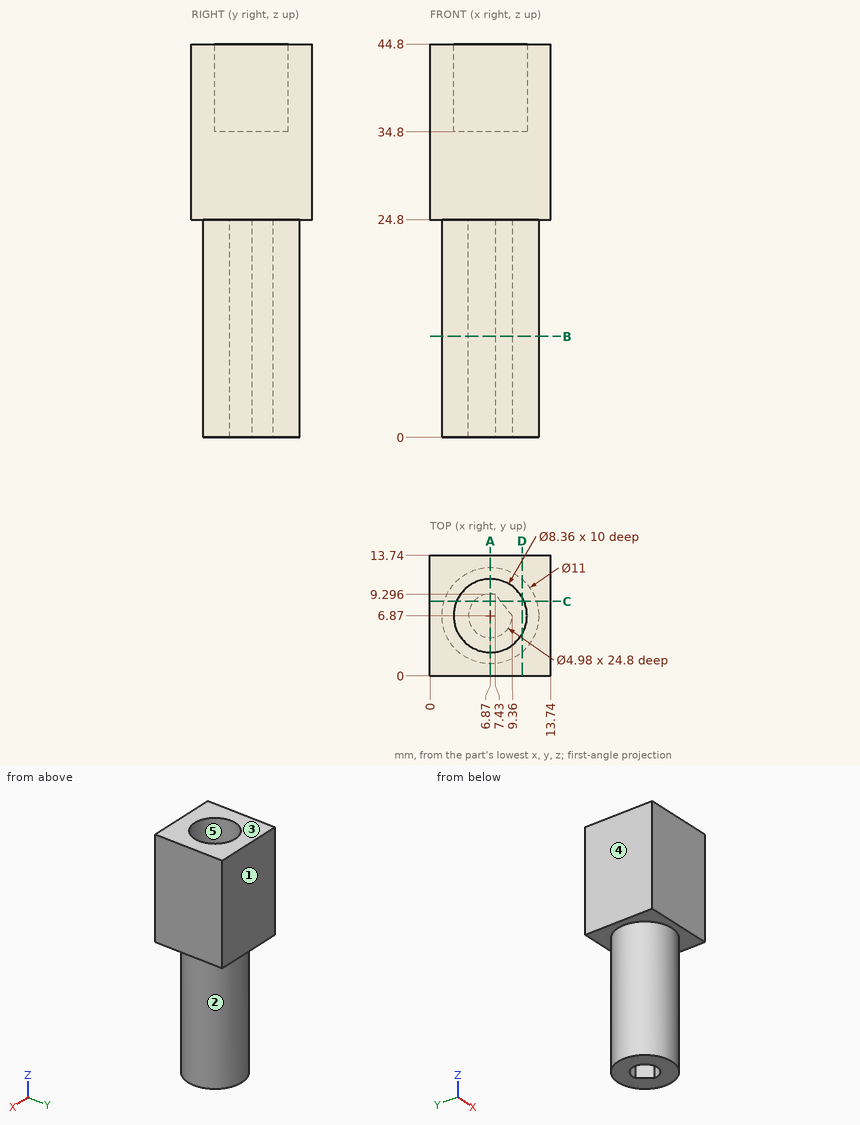
Verification items for this drawing (mm, ordinates from the low corner). A direction names the side the tool comes from. Coordinates: 2 decimals unless noted, no trailing zeros. Order: outer loops, then holes, each group sorted by start corner. A loop starts at its lowest first (then second) coordinate and runs counter-clockwise, first axis right, second up. Notation, with made-up numbers: (27.25, -18.5) -> (85.25, -18.5) arc R8 ccw to (85.25, -3.5) -> close; hole circle Ø10 at (-5.5, 51.25). An arc over 180 degrees is marked (long way). Answer as CSV lines item,"result". Start each with the question number.
1) Cross-section at D-D, the plane x = 10.5. Record the boundary of the cut face in (y, z).
2) Release check for a two-part mould opening along X. For the marked faces 3, 4 and 5 record: released by +X, released by -X, zero draft, split by the parting line, or undercut.
3) Gauge pin test, flat ends, axial feed: pin 1 Ø1.5 at (x, z) = (10.5, 21) entering from -Y (1 decimal); pin 2 Ø5 at (x, z) = (4.5, 16) entering from -Y; pin 3 Ø7.5 at (x, y) = (6.87, 6.87) entering from +Z. Record the tip position at first contact, or that the pin passes through.
4) Cross-section at C-C, the plane y = 8.5. Record the boundary of the cut face in (x, z).
5) Cross-section at A-A, the plane x = 6.87. Record the boundary of the cut face in (y, z).
6) Set-up check for the marked faces 1 and 2: record each of +Z, -Z, +X, -X, +Y, -Y from which the full face is reachable in a straight line by a thin tool's end or side.
7) Cross-section at B-B, the plane z = 11.5. Record the boundary of the cut face in (x, y).
8) Material ranges on L1, parallel to X at y = 6.87, z = 18; L2, parallel to Y at x = 6.87, z = 37.5; L3, parallel to Z at x = 3, y = 8, recorded low to high. Write a range as [from, to].
Conclusion:
1,outline,"(0, 24.8) -> (2.74, 24.8) -> (2.74, 0) -> (11, 0) -> (11, 24.8) -> (13.74, 24.8) -> (13.74, 44.8) -> (8.94, 44.8) -> (8.94, 34.8) -> (4.8, 34.8) -> (4.8, 44.8) -> (0, 44.8) -> close"
2,face 3,"zero draft"
2,face 4,"released by -X"
2,face 5,"undercut"
3,pin 1,"stops at y = 2.2"
3,pin 2,"stops at y = 1.37"
3,pin 3,"stops at z = 34.8"
4,outline,"(0, 24.8) -> (1.62, 24.8) -> (1.62, 0) -> (4.99, 0) -> (4.99, 24.8) -> (8.06, 24.8) -> (8.06, 0) -> (12.12, 0) -> (12.12, 24.8) -> (13.74, 24.8) -> (13.74, 44.8) -> (10.72, 44.8) -> (10.72, 34.8) -> (3.02, 34.8) -> (3.02, 44.8) -> (0, 44.8) -> close"
5,outline,"(0, 24.8) -> (1.37, 24.8) -> (1.37, 0) -> (4.38, 0) -> (4.38, 24.8) -> (9.36, 24.8) -> (9.36, 0) -> (12.37, 0) -> (12.37, 24.8) -> (13.74, 24.8) -> (13.74, 44.8) -> (11.05, 44.8) -> (11.05, 34.8) -> (2.69, 34.8) -> (2.69, 44.8) -> (0, 44.8) -> close"
6,face 1,"+Z, -Z, +X, -X, +Y"
6,face 2,"-Z"
7,outline,"circle Ø11 at (6.87, 6.87); hole (7.43, 9.3) arc R2.49 ccw (long way) to (9.36, 6.87) -> close"
8,L1,"x = [1.37, 4.38], [9.36, 12.37]"
8,L2,"y = [0, 2.69], [11.05, 13.74]"
8,L3,"z = [0, 34.8]"
